Verification items for the finished model (mm, model axes). Coordinates: 2 decimals unless noted, no trailing zeros. Order: outer loops, then holes, each group sorted by start corner. A loop starts at its lowest first (then second) coordinate and runs counter-clockwise, first axis right, second up. Notation, with made-up numbers: M 56,16 L 80,16 A27 ccw 80,48 Z; hole C 42,-14.75 d11. An arc over 180 degrees is marked long. Write item = value, one per line.
```python
from build123d import *

# Parameters (mm, degrees)
SKETCH1_W                      = 203.2
SKETCH1_H                      = 101.6
BOSS_EXTRUDE1_DEPTH            = 6.35
F_1_2_0_5_DIAMETER_HOLE1_D     = 12.7
F_1_2_0_5_DIAMETER_HOLE1_DEPTH = 25.4
F_1_2_0_5_DIAMETER_HOLE1_TIP   = 3.815464931
SKETCH4_R                      = 20.6375
CUT_EXTRUDE1_DEPTH             = 161.50344791
F_3_8_16_TAPPED_HOLE1_D        = 7.9375
F_3_8_16_TAPPED_HOLE1_DEPTH    = 23.8125
F_3_8_16_TAPPED_HOLE1_TIP      = 2.384665582


with BuildPart() as part:
    # Sketch1 → Boss-Extrude1 (new body)
    with BuildSketch(Plane(origin=(0, 0, 0), x_dir=(1, 0, 0), z_dir=(0, 1, 0))):
        with Locations((42.817129402, 18.947595129)):
            Rectangle(SKETCH1_W, SKETCH1_H)
    extrude(amount=BOSS_EXTRUDE1_DEPTH)

    # 1/2 (0.5) Diameter Hole1
    with Locations(Plane(origin=(-33.382870598, 6.35, -18.947595129), x_dir=(0, 0, 1), z_dir=(0, 1, 0))):
        with Locations((0, 0), (0, 152.4)):
            Hole(F_1_2_0_5_DIAMETER_HOLE1_D / 2, depth=F_1_2_0_5_DIAMETER_HOLE1_DEPTH)
            with Locations((0, 0, -(F_1_2_0_5_DIAMETER_HOLE1_DEPTH + F_1_2_0_5_DIAMETER_HOLE1_TIP / 2))):  # 118° drill point
                Cone(0, F_1_2_0_5_DIAMETER_HOLE1_D / 2, F_1_2_0_5_DIAMETER_HOLE1_TIP, mode=Mode.SUBTRACT)

    # Sketch4 → Cut-Extrude1 (cut, through all)
    with BuildSketch(Plane(origin=(0, 6.35, 0), x_dir=(1, 0, 0), z_dir=(0, 1, 0))):
        with Locations(Location((42.817129402, 18.947595129, 0), (0, 0, 270))):
            Circle(SKETCH4_R)
    extrude(amount=-CUT_EXTRUDE1_DEPTH, mode=Mode.SUBTRACT)

    # 3/8-16 Tapped Hole1
    with Locations(Plane(origin=(4.717129402, 6.35, -57.047595129), x_dir=(0, 0, 1), z_dir=(0, 1, 0))):
        with Locations((0, 0), (0, 76.2), (76.2, 76.2), (76.2, 0)):
            Hole(F_3_8_16_TAPPED_HOLE1_D / 2, depth=F_3_8_16_TAPPED_HOLE1_DEPTH)
            with Locations((0, 0, -(F_3_8_16_TAPPED_HOLE1_DEPTH + F_3_8_16_TAPPED_HOLE1_TIP / 2))):  # 118° drill point
                Cone(0, F_3_8_16_TAPPED_HOLE1_D / 2, F_3_8_16_TAPPED_HOLE1_TIP, mode=Mode.SUBTRACT)


solid = part.part
```
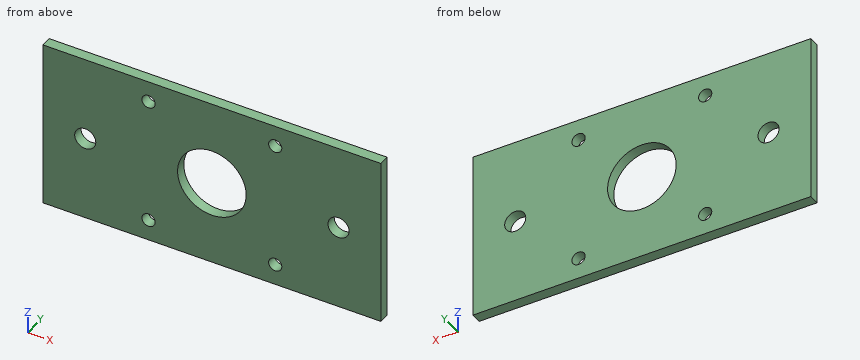
Item 1: Sectioned sample at D-D, the plane y = 5.25. Give the number of separate pieces and of enclosed holes in the cut face, then the cut area to 3 significant figures.
Report:
separate_pieces = 1
enclosed_holes = 7
area = 18,900 mm^2
Item 2: Sectioned sample at A-A, the plane z = -2.5. Enter the section's corners in (x, y).
Report:
outline = M -58.78,0 L 30.35,0 L 30.35,6.35 L -58.78,6.35 Z; M 55.28,0 L 144.42,0 L 144.42,6.35 L 55.28,6.35 Z
Item 3: Scan lines: L1, parallel to X at y = 2.75, z = -60; L2, parallel to X at y = 2, z = -16; L3, parallel to Z at x = 78, y = 5.75. Record each from-to range of solid material in increasing order. Write a range as from..to.
Report:
L1 = -58.78..2.06, 7.37..78.26, 83.57..144.42
L2 = -58.78..-39.01, -27.76..22.39, 63.24..113.39, 124.64..144.42
L3 = -69.75..-59.74, -54.36..16.46, 21.84..31.85
Item 4: Sectioned sample at C-C, the plane x = 30.5. Enter the section's corners in (y, z).
Report:
outline = M 0,-69.75 L 6.35,-69.75 L 6.35,-35.51 L 0,-35.51 Z; M 0,-2.39 L 6.35,-2.39 L 6.35,31.85 L 0,31.85 Z
Item 5: Sectioned sample at B-B, the plane x = 79. Enter the section's corners in (y, z), then the cut area to 3 significant figures.
Report:
outline = M 0,-69.75 L 6.35,-69.75 L 6.35,-60.52 L 0,-60.52 Z; M 0,-53.57 L 6.35,-53.57 L 6.35,15.68 L 0,15.68 Z; M 0,22.63 L 6.35,22.63 L 6.35,31.85 L 0,31.85 Z
area = 557 mm^2
